from build123d import *

# Parameters (mm, degrees)
SKETCH1_R           = 2.5527
BOSS_EXTRUDE1_DEPTH = 3.175


with BuildPart() as part:
    # Sketch1 → Boss-Extrude1 (new body)
    with BuildSketch(Plane(origin=(0, 0, 0), x_dir=(-1, 0, 0), z_dir=(0, 0, -1))):
        with BuildLine():
            Line((-73.66, 394.97), (-113.03, 394.97))
            ThreePointArc((-113.03, 394.97), (-113.928025612, 394.598025612), (-114.3, 393.7))
            Line((-114.3, 393.7), (-114.3, 393.065))
            ThreePointArc((-114.3, 393.065), (-115.043948776, 391.268948776), (-116.84, 390.525))
            Line((-116.84, 390.525), (-179.109843752, 390.525))
            ThreePointArc((-179.109843752, 390.525), (-180.007869365, 390.689047559), (-180.789895835, 391.16))
            ThreePointArc((-180.789895835, 391.16), (-186.240104165, 391.980104165), (-189.23, 387.35))
            Line((-189.23, 387.35), (-189.23, 292.1))
            ThreePointArc((-189.23, 292.1), (-188.486051224, 290.303948776), (-186.69, 289.56))
            Line((-186.69, 289.56), (-176.779113577, 289.56))
            ThreePointArc((-176.779113577, 289.56), (-175.509113577, 289.219704526), (-174.579409051, 288.29))
            ThreePointArc((-174.579409051, 288.29), (-170.18, 285.75), (-165.780590949, 288.29))
            ThreePointArc((-165.780590949, 288.29), (-164.850886423, 289.219704526), (-163.580886423, 289.56))
            Line((-163.580886423, 289.56), (-113.03, 289.56))
            ThreePointArc((-113.03, 289.56), (-111.233948776, 288.816051224), (-110.49, 287.02))
            Line((-110.49, 287.02), (-110.49, 286.258))
            ThreePointArc((-110.49, 286.258), (-109.746051224, 284.461948776), (-107.95, 283.718))
            Line((-107.95, 283.718), (-74.93, 283.718))
            ThreePointArc((-74.93, 283.718), (-73.133948776, 284.461948776), (-72.39, 286.258))
            Line((-72.39, 286.258), (-72.39, 287.02))
            ThreePointArc((-72.39, 287.02), (-71.646051224, 288.816051224), (-69.85, 289.56))
            Line((-69.85, 289.56), (-5.329113577, 289.56))
            ThreePointArc((-5.329113577, 289.56), (-4.059113577, 289.219704526), (-3.129409051, 288.29))
            ThreePointArc((-3.129409051, 288.29), (2.584800749, 285.923096802), (6.35, 290.83))
            Line((6.35, 290.83), (6.35, 380.165795103))
            ThreePointArc((6.35, 380.165795103), (6.816098684, 381.632264787), (8.043333333, 382.560530069))
            ThreePointArc((8.043333333, 382.560530069), (10.729754791, 389.923742018), (2.989895835, 391.16))
            ThreePointArc((2.989895835, 391.16), (2.207869365, 390.689047559), (1.309843752, 390.525))
            Line((1.309843752, 390.525), (-69.85, 390.525))
            ThreePointArc((-69.85, 390.525), (-71.646051224, 391.268948776), (-72.39, 393.065))
            Line((-72.39, 393.065), (-72.39, 393.7))
            ThreePointArc((-72.39, 393.7), (-72.761974388, 394.598025612), (-73.66, 394.97))
        make_face()
        with Locations(Location((-184.15, 387.35, 0), (0, 0, 180))):
            Circle(SKETCH1_R, mode=Mode.SUBTRACT)
        with Locations(Location((-107.95, 387.35, 0), (0, 0, 180))):
            Circle(SKETCH1_R, mode=Mode.SUBTRACT)
        with Locations(Location((-82.55, 387.35, 0), (0, 0, 180))):
            Circle(SKETCH1_R, mode=Mode.SUBTRACT)
        with Locations(Location((1.27, 290.83, 0), (0, 0, 180))):
            Circle(SKETCH1_R, mode=Mode.SUBTRACT)
        with Locations(Location((-104.14, 291.1475, 0), (0, 0, 180))):
            Circle(SKETCH1_R, mode=Mode.SUBTRACT)
        with Locations(Location((-78.74, 291.1475, 0), (0, 0, 180))):
            Circle(SKETCH1_R, mode=Mode.SUBTRACT)
        with Locations(Location((6.35, 387.35, 0), (0, 0, 180))):
            Circle(SKETCH1_R, mode=Mode.SUBTRACT)
        with Locations(Location((-170.18, 290.83, 0), (0, 0, 180))):
            Circle(SKETCH1_R, mode=Mode.SUBTRACT)
        with BuildLine():
            Line((-72.39, 378.46), (-72.39, 381.635))
            ThreePointArc((-72.39, 381.635), (-71.646051224, 383.431051224), (-69.85, 384.175))
            Line((-69.85, 384.175), (-2.54, 384.175))
            ThreePointArc((-2.54, 384.175), (-0.743948776, 383.431051224), (0, 381.635))
            Line((0, 381.635), (0, 298.45))
            ThreePointArc((0, 298.45), (-0.743948776, 296.653948776), (-2.54, 295.91))
            Line((-2.54, 295.91), (-180.34, 295.91))
            ThreePointArc((-180.34, 295.91), (-182.136051224, 296.653948776), (-182.88, 298.45))
            Line((-182.88, 298.45), (-182.88, 380.750886423))
            ThreePointArc((-182.88, 380.750886423), (-182.539704526, 382.020886423), (-181.61, 382.950590949))
            ThreePointArc((-181.61, 382.950590949), (-181.185264253, 383.224864614), (-180.789895835, 383.54))
            ThreePointArc((-180.789895835, 383.54), (-180.007869365, 384.010952441), (-179.109843752, 384.175))
            Line((-179.109843752, 384.175), (-116.84, 384.175))
            ThreePointArc((-116.84, 384.175), (-115.043948776, 383.431051224), (-114.3, 381.635))
            Line((-114.3, 381.635), (-114.3, 378.46))
            ThreePointArc((-114.3, 378.46), (-113.928025612, 377.561974388), (-113.03, 377.19))
            Line((-113.03, 377.19), (-73.66, 377.19))
            ThreePointArc((-73.66, 377.19), (-72.761974388, 377.561974388), (-72.39, 378.46))
        make_face(mode=Mode.SUBTRACT)
    extrude(amount=-BOSS_EXTRUDE1_DEPTH)


solid = part.part
Input: part model. Units: mm. Frame: model coordinates. Round coordinates to 2 decimals unless told otherwise and drop trailing zeros. Order: outer loops, then holes, each group sorted by start corner. A loop starts at its lowest first (then second) coordinate and runs counter-clockwise, first axis right, second up. Notation, with made-up numbers: (55, -19) - (113, -19) arc R7 cw to (113, -10) - close; hole circle Ø4 at (87, 48.25). An arc over 180 degrees is marked (long way). Answer as a JSON object with one key per item and string values. Group by question number.
(1) Pin query (flat end, axial travel): P1, Ø1, axis at x = 146.5, z = 1, coming from the -Y side; P2, Ø1.6, axis at x = 144, z = 1, coming from the +Y side (3 decimals); P3, Ø1.5, axis at y = 344.5, z = 0.5, coming from the -X side; P4, Ø6, axis at x = 104.14, y = 291.15, coming from the +Z side (3 decimals). Return the tip coordinate at first contact, or that it passes through.
(2) Draft query along Y for faces 1 (the face through (-10.8, 389.8, 1.6)), 2 (the face through (83.922, 385.198, 1.565)), 3 (the face through (104, 381, 0)). Return one class per face: released by +Y, released by -Y, zero draft, split by the parting line, or undercut.
(3) Cut plane B-B (x = 99.5). Return loops of the section in (y, z) (3 decimals), then the cut area to 3 significant figures.
(4) Cut plane C-C (x = 18.5). Return loops of the section in (y, z) (3 decimals).
(5) Cut plane D-D (z = 1.9). Count the separate pieces of the cut face and the enclosed holes in it, then the cut area to 3 significant figures.
(6) Cut plane A-A (x = 170.18). Return loops of the section in (y, z) (3 decimals).
(7) Material intervals for probe 1 along X at (y, z) = (379.5, 2.25); probe 2 along Y at (x, z) = (104.14, 1.8); probe 3 along X at (y, z) = (387, 2.3), sorted ascending. Write a range as from..to.
Here are the results:
{
 "1": {"P1": "stops at y = 289.56", "P2": "stops at y = 390.525", "P3": "stops at x = -6.35", "P4": "stops at z = 3.175"},
 "2": {"face 1": "split by the parting line", "face 2": "undercut", "face 3": "zero draft"},
 "3": {"outline": "(283.718, 0) - (295.91, 0) - (295.91, 3.175) - (283.718, 3.175) - close; (377.19, 0) - (394.97, 0) - (394.97, 3.175) - (377.19, 3.175) - close", "area": "95.2 mm^2"},
 "4": {"outline": "(289.56, 0) - (295.91, 0) - (295.91, 3.175) - (289.56, 3.175) - close; (384.175, 0) - (390.525, 0) - (390.525, 3.175) - (384.175, 3.175) - close"},
 "5": {"separate pieces": "1", "enclosed holes": "9", "area": "4,270 mm^2"},
 "6": {"outline": "(285.75, 0) - (288.277, 0) - (288.277, 3.175) - (285.75, 3.175) - close; (293.383, 0) - (295.91, 0) - (295.91, 3.175) - (293.383, 3.175) - close; (384.175, 0) - (390.525, 0) - (390.525, 3.175) - (384.175, 3.175) - close"},
 "7": {"probe 1": "x = -6.35..0, 72.39..114.3, 182.88..189.23", "probe 2": "y = 283.72..288.59, 293.7..295.91, 377.19..394.97", "probe 3": "x = -11.42..-8.88, -3.82..80.02, 85.08..105.42, 110.48..181.62, 186.68..189.23"}
}
